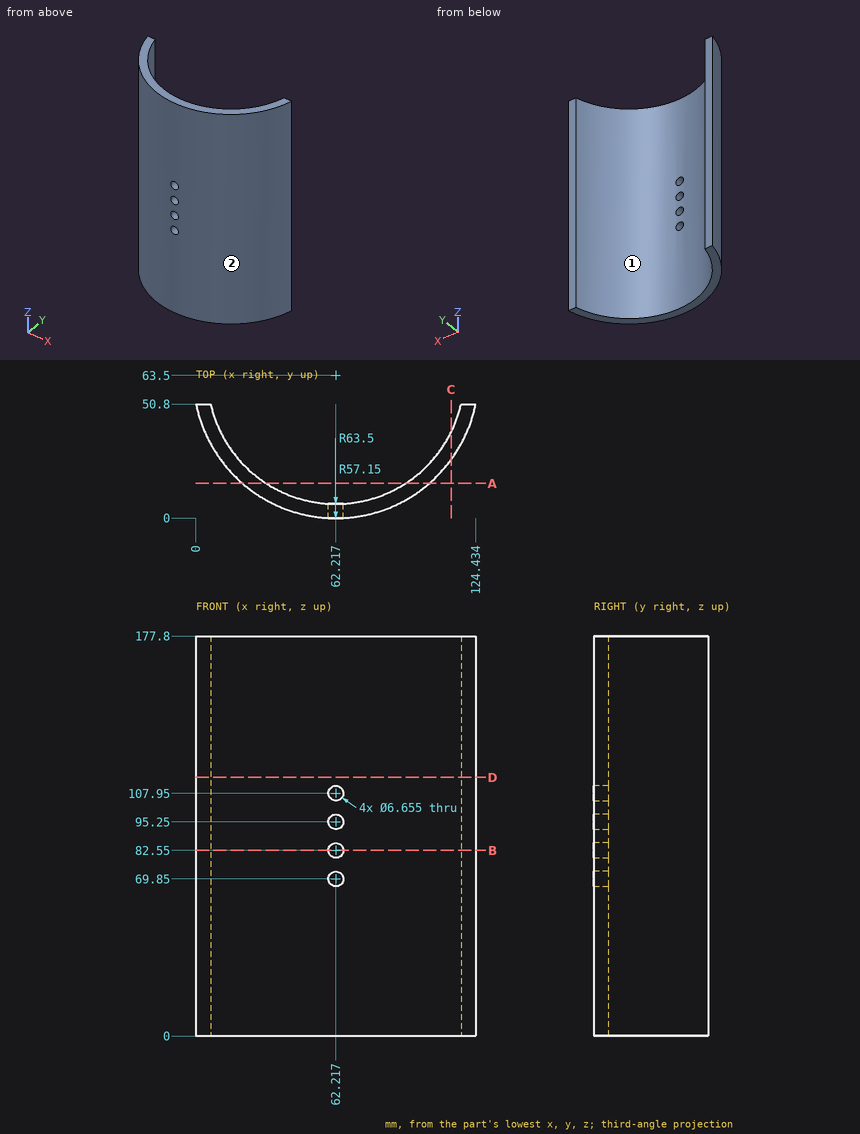
Geometry check sheet. Reference: drawing and pictorial views, mm from the part's lowest x, y, z. Round coordinates to 2 decimals unless told otherwise and drop trailing zeros. Loops run counter-clockwise (first coordinate to the right, second up) from the corner with the lowest first, then second, coordinate; pieces in that order, holes last. Notation, with made-up numbers: (-24, 35) - (-6, 35) arc R18 cw to (-6, 57) - close; hole circle Ø7 at (-7, 29.5). An arc over 180 degrees is marked (long way). One line per question, with ' | ' between items. Start each with the question number.
1. Cross-section at A-A on y = 15.5. Record the cut outline in (x, z) (3 decimals).
2. Draft check along X on the marked faces 1 and 2. Enter one of: released by +X, released by -X, zero draft, split by the parting line, or undercut.
3. Cross-section at B-B on z = 82.55. Record the cut outline in (x, y), then the cut area to 3 significant figures.
4. Cross-section at D-D on z = 115. Record the cut outline in (x, y), then the cut area to 3 significant figures.
5. Scan lines: line 1 (X direction, y = 5, z = 107.95) (1 decimal); line 2 (X direction, y = 47.5, z = 29.5); line 3 (Y direction, x = 18.5, z = 87) (1 decimal). Record each from-to range of solid material in increasing order. Write a range as [from, to].
6. Depth check by flat-ended pin: pin 1 (12 mm diameter, centred on x = 108, z = 86.5, fed in from +Y); pin 2 (7.5 mm diameter, centred on x = 62.22, z = 107.95, fed in from -Y); pin 3 (12 mm diameter, centred on y = 8.5, z = 21.5, fed in from -X); pin 4 (12 mm diameter, centred on x = 16.5, z = 146.5, fed in from -Y). Enter the tip coordinate at first touch or a pass-through.
7. Cross-section at C-C on x = 113.5. Record the cut outline in (y, z).
Taken from the geometry:
1) outline: (20.645, 0) - (31.199, 0) - (31.199, 177.8) - (20.645, 177.8) - close; (93.235, 0) - (103.789, 0) - (103.789, 177.8) - (93.235, 177.8) - close
2) face 1: undercut | face 2: split by the parting line
3) outline: (0, 50.8) arc R63.5 ccw to (58.89, 0.09) - (58.89, 6.45) arc R57.15 cw to (6.5, 50.8) - close; (65.54, 0.09) arc R63.5 ccw to (124.43, 50.8) - (117.94, 50.8) arc R57.15 cw to (65.54, 6.45) - close | area: 999 mm²
4) outline: (0, 50.8) arc R63.5 ccw to (124.43, 50.8) - (117.94, 50.8) arc R57.15 cw to (6.5, 50.8) - close | area: 1,040 mm²
5) line 1: [37.5, 58.9], [65.5, 86.9] | line 2: [0.77, 7.35], [117.08, 123.67] | line 3: [17.4, 26.7]
6) pin 1: y = 39.32 | pin 2: y = 0 | pin 3: x = 21.83 | pin 4: y = 13.95
7) outline: (26.05, 0) - (38.28, 0) - (38.28, 177.8) - (26.05, 177.8) - close
